For this review, take the finished solid that the model builds, in its own axes (mm). A direction names the side the tool comes from. Round coordinates to 2 decimals unless told otherwise and drop trailing zeros. Write each loop counter-clockwise with the first axis right and the second up, starting at its lowest first coordinate (ties: lowest second). Pieces come first, ordered by that corner, then holes. Notation, with made-up numbers: (85, 6.25) -> (89, 6.25) arc R31 cw to (89, 34.25) -> close; hole circle Ø3 at (19, 7). An arc over 180 degrees is marked (long way). Answer as CSV lines item,"result". Start each with the question number.
Item 1: Wall thickness on probe 1 along Z at (x, y) = (6.75, 16.5); probe 2 along X at (y, z) = (16.5, 0.7); probe 3 along Y at (x, z) = (4.5, 0.1): over which ranges is each line inside the solid? List them lowest first. Write a range as from..to.
Item 2: Mouldability with a two-part tool opening along Y and no side actions: class faces 1 (the cylindrical face through (0.1, 19.5, 0.7)), 2 (the flat face through (-5, 4, 1)), 3 (the flat face through (-4, 1, 0)) as +Y half, -Y half, draft (parallel to the pull), parting line (faces both ways), or undercut.
Item 3: Take a section at D-D on x = 8.25. Give the boundary of the cut face in (y, z).
Item 4: For pin 1 Ø1.7 at (x, y) = (5, 16.5) entering from -Z, flat-tipped, find the tip position at first contact; note if it passes through.
Item 5: Take a section at B-B on y = 17. Give the boundary of the cut face in (x, z).
Item 6: Take a section at C-C on x = -6.75. Give the boundary of the cut face in (y, z).
Item 7: Take a section at A-A on z = 0.6. Count the separate pieces of the cut face and the enclosed holes in it, then the cut area to 3 significant figures.
Item 8: Machinability: for faces 4 (the flat face through (5.86, 0.6, 0.4)), 5 (the flat face through (-0.71, 3.7, 0.5)), 6 (the flat face through (6, 17, 1.2)), 7 (the flat face through (0, 0, 1)), 8 (the flat face through (0, 10, 0)), which of the approach directions +Z, -Z, +X, -X, +Y, -Y give a long, thin tool a straight path to every point of the face, cutting with its end or side? Answer none if there is none.
```python
from build123d import *

# Parameters (mm, degrees)
F1_DEPTH  = 1.5
F2_R      = 1.7
F3_DEPTH  = 1.2
F5_DEPTH  = 1
F6_W      = 0.8
F6_H      = 2.7
F7_DEPTH  = 0.3
F8_W      = 0.55
F8_H      = 0.9
F9_DEPTH  = 1.2
F10_W     = 0.3
F10_H     = 0.3
F10_W_2   = 0.0500000367
F10_H_2   = 0.05
F10_W_3   = 0.0499999633
F11_DEPTH = 1


with BuildPart() as f1:
    # F0 (on Top) → F1 (new body)
    with BuildSketch(Plane.XY):
        with BuildLine():
            Line((-8.9560451977, 14.5), (-9.21, 0))
            Line((-9.21, 0), (9.21, 0))
            Line((9.21, 0), (8.9560451977, 14.5))
            ThreePointArc((8.9560451977, 14.5), (8.8000416812, 15.4975744796), (8.9210169492, 16.5))
            Line((8.9210169492, 16.5), (8.9, 17.7))
            Line((8.9, 17.7), (-8.9, 17.7))
            Line((-8.9, 17.7), (-8.9210169492, 16.5))
            ThreePointArc((-8.9210169492, 16.5), (-8.8000416812, 15.4975744796), (-8.9560451977, 14.5))
        make_face()
        with BuildLine():
            ThreePointArc((8.9, 17.7), (0, 19.5), (-8.9, 17.7))
            Line((-8.9, 17.7), (8.9, 17.7))
        make_face()
    extrude(amount=F1_DEPTH)

    # F2 (on Top) → F3 (cut)
    with BuildSketch(Plane.XY):
        with Locations((5.6, 17)):
            Circle(F2_R)
        with Locations((-5.6, 17)):
            Circle(F2_R)
    extrude(amount=F3_DEPTH, mode=Mode.SUBTRACT)

    # F4 (on face) → F5 (cut)
    with BuildSketch(Plane(origin=(0, 0, 0), x_dir=(1, 0, 0), z_dir=(0, 0, -1))):
        Polygon((-9.1276836158, -4.7), (-0.71, -4.7), (-0.71, -2.7), (-9.1627118644, -2.7), align=None)
    extrude(amount=-F5_DEPTH, mode=Mode.SUBTRACT)

    # F6 (on face) → F7 (cut)
    with BuildSketch(Plane(origin=(0, 0, 0), x_dir=(1, 0, 0), z_dir=(0, 0, -1))):
        with Locations((-1.71, -1.35)):
            Rectangle(F6_W, F6_H)
        with Locations((-5.81, -1.35)):
            Rectangle(F6_W, F6_H)
    extrude(amount=-F7_DEPTH, mode=Mode.SUBTRACT)

    # F8 (on face) → F9 (cut)
    with BuildSketch(Plane.XZ):
        with Locations((6.135, 0.45)):
            Rectangle(F8_W, F8_H)
        with Locations((5.285, 0.45)):
            Rectangle(F8_W, F8_H)
        with Locations((1.185, 0.45)):
            Rectangle(F8_W, F8_H)
        with Locations((2.035, 0.45)):
            Rectangle(F8_W, F8_H)
    extrude(amount=-F9_DEPTH, mode=Mode.SUBTRACT)

    # F10 (on face) → F11 (cut)
    with BuildSketch(Plane.XZ):
        with Locations((1.6100000367, 1.05)):
            Rectangle(F10_W, F10_H)
        with Locations((1.7850000184, 0.875)):
            Rectangle(F10_W_2, F10_H_2)
        with Locations((1.61, 0.875)):
            Rectangle(F10_W, F10_H_2)
        with Locations((1.4350000184, 0.875)):
            Rectangle(F10_W_3, F10_H_2)
        Polygon((1.4100000367, 1.25), (1.4100000367, 0.9), (1.46, 0.9), (1.4600000367, 1.2), (1.7600000367, 1.2), (1.7600000367, 0.9), (1.8100000367, 0.9), (1.8100000367, 1.25), align=None)
        Polygon((5.5100000367, 1.25), (5.5100000367, 0.9), (5.56, 0.9), (5.5600000367, 1.2), (5.8600000367, 1.2), (5.8600000367, 0.9), (5.9100000367, 0.9), (5.9100000367, 1.25), align=None)
        with Locations((5.7100000367, 1.05)):
            Rectangle(F10_W, F10_H)
        with Locations((5.71, 0.875)):
            Rectangle(F10_W, F10_H_2)
        with Locations((5.8850000184, 0.875)):
            Rectangle(F10_W_2, F10_H_2)
        with Locations((5.5350000184, 0.875)):
            Rectangle(F10_W_3, F10_H_2)
    extrude(amount=-F11_DEPTH, mode=Mode.SUBTRACT)


solid = f1.part
```
Output values:
1,probe 1,"z = 1.2..1.5"
1,probe 2,"x = -8.92..-7.22, -3.98..3.98, 7.22..8.92"
1,probe 3,"y = 0..15.7, 18.3..19.05"
2,face 1,"+Y half"
2,face 2,"undercut"
2,face 3,"draft"
3,outline,"(0, 0) -> (17.96, 0) -> (17.96, 1.5) -> (0, 1.5) -> close"
4,pin 1,"stops at z = 1.2"
5,outline,"(-8.91, 0) -> (-7.3, 0) -> (-7.3, 1.2) -> (-3.9, 1.2) -> (-3.9, 0) -> (3.9, 0) -> (3.9, 1.2) -> (7.3, 1.2) -> (7.3, 0) -> (8.91, 0) -> (8.91, 1.5) -> (-8.91, 1.5) -> close"
6,outline,"(0, 0) -> (2.7, 0) -> (2.7, 1) -> (4.7, 1) -> (4.7, 0) -> (15.75, 0) -> (15.75, 1.2) -> (18.25, 1.2) -> (18.25, 0) -> (18.48, 0) -> (18.48, 1.5) -> (0, 1.5) -> close"
7,separate pieces,"1"
7,enclosed holes,"2"
7,area,"304 mm^2"
8,face 4,"-Z, -Y"
8,face 5,"-Z, -X"
8,face 6,"-Z"
8,face 7,"+Z, -Z, +X, -X, -Y"
8,face 8,"-Z, +X, -X, +Y, -Y"
